Design review of the part built by this model. Coordinates are the model's own, in mm. Give positions to 0.01 mm unless a question says otherwise; leave off trailing zeros. Order: outer loops, then holes, each group sorted by start corner. A loop starts at its lowest first (then second) coordinate and runs counter-clockwise, first axis right, second up. Notation, with made-up numbers: M 43,-34 L 48,-34 A22 ccw 48,2 Z; hole C 36.5,44 d11. An arc over 180 degrees is marked long. Put each result on its own line as item: value. Start each with the question number.
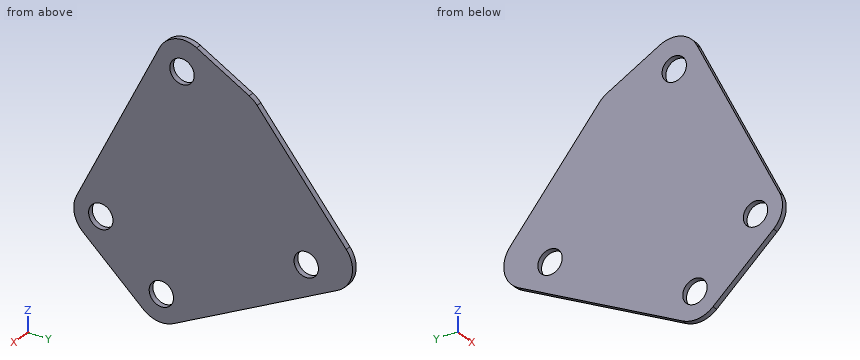
from build123d import *

# Parameters (mm, degrees)
SKETCH1_R           = 2.25
BOSS_EXTRUDE1_DEPTH = 0.5


with BuildPart() as part:
    # Sketch1 → Boss-Extrude1 (new body, symmetric)
    with BuildSketch(Plane(origin=(0, 0, 0), x_dir=(0, 0, -1), z_dir=(1, 0, 0))):
        with BuildLine():
            Line((-2.842316383, -4.169011752), (27.763932023, -19.472135955))
            ThreePointArc((27.763932023, -19.472135955), (30.93796237, -19.911234732), (33.726779962, -18.333333333))
            Line((33.726779962, -18.333333333), (43.726779962, -7.152993446))
            ThreePointArc((43.726779962, -7.152993446), (44.957632334, -4.469184277), (44.459693025, -1.558877478))
            Line((44.459693025, -1.558877478), (29.09925887, 28.74161228))
            ThreePointArc((29.09925887, 28.74161228), (25.660151825, 31.375561942), (21.454986898, 30.335496549))
            Line((21.454986898, 30.335496549), (1.506318758, 13.854666903))
            ThreePointArc((1.506318758, 13.854666903), (0.835117993, 13.183231504), (0.302931344, 12.397029665))
            Line((0.302931344, 12.397029665), (-4.994214766, 2.700153867))
            ThreePointArc((-4.994214766, 2.700153867), (-5.377602176, -1.19159423), (-2.842316383, -4.169011752))
        make_face()
        with Locations((30, -15)):
            Circle(SKETCH1_R, mode=Mode.SUBTRACT)
        with Locations((40, -3.819660113)):
            Circle(SKETCH1_R, mode=Mode.SUBTRACT)
        Circle(SKETCH1_R, mode=Mode.SUBTRACT)
        with Locations((26.435304192, 22.938498039)):
            Circle(SKETCH1_R, mode=Mode.SUBTRACT)
    extrude(amount=BOSS_EXTRUDE1_DEPTH, both=True)


solid = part.part
1. Consider section B-B on z = -30.5. Give the boundary of the cut face in (x, y), then the cut area to 3 significant figures.
2. Consider section D-D on z = -8.5. Give the boundary of the cut face in (x, y), then the cut area to 3 significant figures.
3. Consider section C-C on x = -0.15. Give the boundary of the cut face in (y, z).
4. Consider section A-A on y = -15. Give the boundary of the cut face in (x, z).
5. Insertion check: pin 1 (6 mm diameter, centred on y = 22.94, z = -26.44, fed in from +X). The pin has a flat end and moves straight along its axis. Give the tip position at first contact, or say it passes through.
6. To check wall thickness, follow probe 1 along Z at (x, y) = (0.3, 21.5); probe 2 along Y at (x, z) = (0.05, -40); probe 3 along Y at (x, z) = (0.4, -1). State the ranges of each line that lie inside material, in increasing order.
Returned:
1. outline: M -0.5,-19.97 L 0.5,-19.97 L 0.5,-17.19 L -0.5,-17.19 Z; M -0.5,-12.81 L 0.5,-12.81 L 0.5,25.98 L -0.5,25.98 Z
1. area: 41.6 mm2
2. outline: M -0.5,-9.84 L 0.5,-9.84 L 0.5,19.63 L -0.5,19.63 Z
2. area: 29.5 mm2
3. outline: M -19.47,-27.76 A5 ccw -18.33,-33.73 L -7.15,-43.73 A5 ccw -1.56,-44.46 L 28.74,-29.1 A5 ccw 30.34,-21.45 L 13.85,-1.51 A5 ccw 12.4,-0.3 L 2.7,4.99 A5 ccw -4.17,2.84 Z; hole C -15,-30 d4.5; hole C -3.82,-40 d4.5; hole C 0,0 d4.5; hole C 22.94,-26.44 d4.5
4. outline: M -0.5,-36.71 L 0.5,-36.71 L 0.5,-32.25 L -0.5,-32.25 Z; M -0.5,-27.75 L 0.5,-27.75 L 0.5,-18.82 L -0.5,-18.82 Z
5. pin 1: stops at x = 0.5
6. probe 1: z = -32.77 to -28.17, -24.71 to -10.76
6. probe 2: y = -11.32 to -6.07, -1.57 to 7.24
6. probe 3: y = -6.09 to -2.02, 2.02 to 13.37
